Answer from the drawing. Dimensions are ordinates in mm from the lowest x, y and z of the part. Round coordinates to 2 decimals unless told otherwise and drop trailing zeros. Order: outer loops, then holes, each group sorted by start corner. A loop starts at its lowest first (then second) coordinate and runs counter-clockwise, first axis right, second up. Notation, with made-up numbers: (-39, -6) - (17, -6) arc R26 cw to (17, 9) - close; hole circle Ø4 at (24, 18.25). An arc over 180 degrees is marked (long way). One line per question, with ' | ' between items. Start each with the question number.
1) Straight lines are drawn through the part: line 1 (Z direction, x = 6.4, y = 12); line 2 (Y direction, x = 6.5, z = 12); line 3 (X direction, y = 10.25, z = 31). For each, find the intervals that lie inside material, in ascending order. Write a range as from..to.
2) The part is cut by section C-C, the plane y = 5. Give the vertices of the cut face in (x, z), plus the area to 3 significant figures.
3) The part is cut by section A-A, the plane x = 2.5. Give the vertices of the cut face in (y, z) (1 decimal), plus the area to 3 significant figures.
4) The part is cut by section B-B, the plane y = 12. Give the vertices of the cut face in (x, z), plus the area to 3 significant figures.
5) Flat-ended cylindrical pins translate along their axes: pin 1 (3 mm diameter, centred on x = 4, z = 44.5, fed in from +Y); pin 2 (12 mm diameter, centred on y = 14, z = 47.5, fed in from +X); pin 3 (1 mm diameter, centred on x = 4.5, y = 10, fed in from -Z). Find the tip coordinate at first contact, or state that the pin passes through.
6) The mould has two halves that part along Y. Classify the marked faces 1, 2 and 3: pulls with the +Y half, pulls with the -Y half, needs draft (parallel to the pull), parting line crosses it, or undercut.
7) The part is cut by section D-D, the plane z = 16. Give the vertices of the cut face in (x, y).
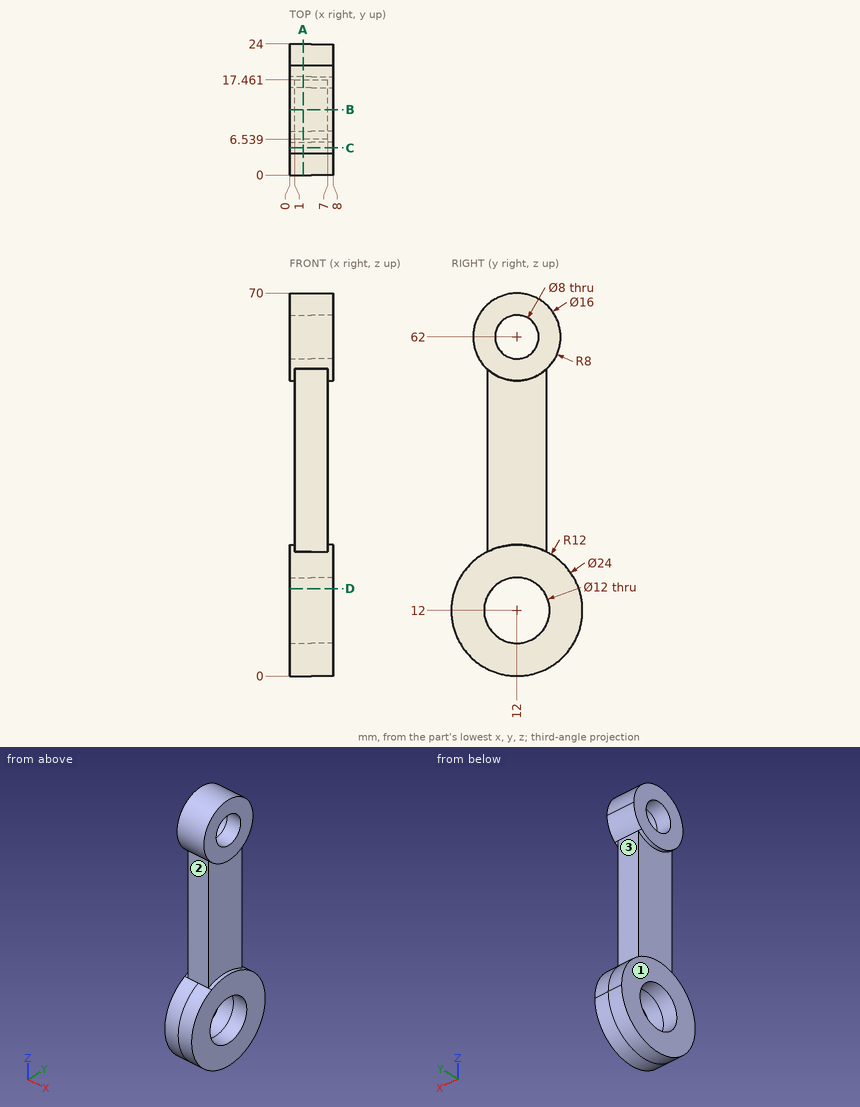
Values:
1) line 1: z = 0..6, 18..58, 66..70 | line 2: y = 0..6, 18..24 | line 3: x = 1..7
2) outline: (0, 2.25) - (8, 2.25) - (8, 21.75) - (0, 21.75) - close; (0, 58.13) - (8, 58.13) - (8, 65.87) - (0, 65.87) - close | area: 218 mm^2
3) outline: (6.5, 22.7) arc R12 ccw (long way) to (17.5, 22.7) - (17.5, 56.2) arc R8 ccw (long way) to (6.5, 56.2) - close; hole circle Ø12 at (12, 12); hole circle Ø8 at (12, 62) | area: 830 mm^2
4) outline: (0, 0) - (8, 0) - (8, 6) - (0, 6) - close; (0, 18) - (8, 18) - (8, 24) - (7, 24) - (7, 54) - (8, 54) - (8, 58) - (0, 58) - (0, 54) - (1, 54) - (1, 24) - (0, 24) - close; (0, 66) - (8, 66) - (8, 70) - (0, 70) - close | area: 340 mm^2
5) pin 1: stops at y = 17.46 | pin 2: stops at x = 7 | pin 3: stops at z = 0.09
6) face 1: needs draft | face 2: pulls with the -Y half | face 3: pulls with the +Y half
7) outline: (0, 0.69) - (8, 0.69) - (8, 7.53) - (0, 7.53) - close; (0, 16.47) - (8, 16.47) - (8, 23.31) - (0, 23.31) - close
